Part model, mm, in its own coordinate system. Coordinates: 2 decimals unless noted, no trailing zeros. Order: outer loops, then holes, each group sorted by start corner. A loop starts at its lowest first (then second) coordinate and runs counter-clockwise, first axis right, second up. Notation, with made-up numbers: (-8.75, -13) - (13.25, -13) arc R25 cw to (13.25, -1) - close; hole circle Ø8 at (65.5, -7.5). An arc over 180 degrees is marked (long way). Use a Markdown table: item, result. Add a question column.
1) Saw through at C-C on z = 2.55. List the corners of the cut face in (x, y).
2) Two-plate mould, pull along X, no slides. Class faces 1 (the face through (-9.498, -0.088, 1.565)), 2 (the face through (15, 0, 2)), 3 (the face through (0, 0, 3.175)): +X half, -X half, draft (parallel to the pull), parting line (faces both ways), or undercut.
3) Saw through at A-A on x = 7.5. List the corners of the cut face in (y, z) (3 decimals), then the cut area to 3 significant figures.
4) Saw through at B-B on y = -1.25. List the corners of the cut face in (x, z) (3 decimals).
5) Saw through at D-D on y = 0.5. List the corners of the cut face in (x, z) (1 decimal).
6) Drop a flat-ended pin along its axis: P1, Ø3, axis at x = 4.5, y = -2, coming from the -Z side. Give the stop position or say it passes through.
7) Wall check: L1, parallel to X at y = 0, z = 2.4; L2, parallel to Y at x = -7.5, z = 1.85; L3, parallel to X at y = 1.75, z = 2.95. Give the ranges that are in metal, low to high. Write a range as [from, to].
Autodesk Inventor part; units mm, degrees
ref_plane "YZ Plane" through (0, 0, 0) normal (1, 0, 0) x (0, 1, 0)
ref_plane "XZ Plane" through (0, 0, 0) normal (0, 1, 0) x (-1, 0, 0)
ref_plane "XY Plane" through (0, 0, 0) normal (0, 0, 1) x (1, 0, 0)
sketch "Sketch1" plane through (0, 0, 0) normal (0, 0, 1) x (1, 0, 0)
  line L0 (15, -7.5) -> (-15, -7.5)
  line L1 (-15, -7.5) -> (-15, 7.5)
  line L2 (-15, 7.5) -> (15, 7.5)
  line L3 (15, 7.5) -> (15, -7.5)
  line L4 (15, -7.5) -> (-15, 7.5) construction
  line L5 (-15, -7.5) -> (15, 7.5) construction
  circle A0 centre (-7.5, 0) radius 2
  circle A1 centre (7.5, 0) radius 2
  line L6 (-21, 0) -> (21, 0)
  line L7 (0, -10.5) -> (0, 10.5)
  line L8 (-7.5, 0) -> (7.5, 0)
  point P0 (0, 0)
  point P1 (0, 0)
  dimension "d10" = 30
  dimension "d11" = 15
  dimension "d12" = 4
  dimension "d13" = 15
extrude "Extrusion1" add sketch "Sketch1" along normal blind 3.175 contours L0 L7 L6 A1 L3 | L0 L1 L6 A0 L7 | L6 A1 L7 L2 L3 | L6 A0 L1 L2 L7
properties part number "soportes celda de carga"
Results are:
| question | item | result |
|---|---|---|
| 1 | outline | (-15, -7.5) - (15, -7.5) - (15, 7.5) - (-15, 7.5) - close; hole circle Ø4 at (-7.5, 0); hole circle Ø4 at (7.5, 0) |
| 2 | face 1 | undercut |
| 2 | face 2 | +X half |
| 2 | face 3 | draft |
| 3 | outline | (-7.5, 0) - (-2, 0) - (-2, 3.175) - (-7.5, 3.175) - close; (2, 0) - (7.5, 0) - (7.5, 3.175) - (2, 3.175) - close |
| 3 | area | 34.9 mm2 |
| 4 | outline | (-15, 0) - (-9.061, 0) - (-9.061, 3.175) - (-15, 3.175) - close; (-5.939, 0) - (5.939, 0) - (5.939, 3.175) - (-5.939, 3.175) - close; (9.061, 0) - (15, 0) - (15, 3.175) - (9.061, 3.175) - close |
| 5 | outline | (-15, 0) - (-9.4, 0) - (-9.4, 3.2) - (-15, 3.2) - close; (-5.6, 0) - (5.6, 0) - (5.6, 3.2) - (-5.6, 3.2) - close; (9.4, 0) - (15, 0) - (15, 3.2) - (9.4, 3.2) - close |
| 6 | P1 | z = 0 |
| 7 | L1 | [-15, -9.5], [-5.5, 5.5], [9.5, 15] |
| 7 | L2 | [-7.5, -2], [2, 7.5] |
| 7 | L3 | [-15, -8.47], [-6.53, 6.53], [8.47, 15] |
